```python
from build123d import *

# Parameters (mm, degrees)
SKETCH_1_R          = 20
SKETCH_1_R_2        = 2.015
SKETCH_1_R_3        = 7.5
SKETCH_1_R_4        = 1.6
EXTRUDE_1_DEPTH     = 6
SKETCH_2_W          = 14.17824661
SKETCH_2_H          = 4
CUT_EXTRUDE_1_DEPTH = 10
FILLET_1_R          = 1


with BuildPart() as part:
    # 草图1 → 凸台-拉伸1 (new body)
    with BuildSketch(Plane(origin=(0, 0, 0), x_dir=(1, 0, 0), z_dir=(0, 1, 0))):
        with Locations(Location((0, 0, 0), (0, 0, 270))):
            Circle(SKETCH_1_R)
        with Locations(Location((0, -12.15, 0), (0, 0, 270))):
            Circle(SKETCH_1_R_2, mode=Mode.SUBTRACT)
        with Locations(Location((10.522208656, 6.075, 0), (0, 0, 270))):
            Circle(SKETCH_1_R_2, mode=Mode.SUBTRACT)
        with Locations(Location((-10.522208656, 6.075, 0), (0, 0, 270))):
            Circle(SKETCH_1_R_2, mode=Mode.SUBTRACT)
        with Locations(Location((0, 0, 0), (0, 0, 270))):
            Circle(SKETCH_1_R_3, mode=Mode.SUBTRACT)
        with Locations(Location((-11.691342951, -6.75, 0), (0, 0, 270))):
            Circle(SKETCH_1_R_4, mode=Mode.SUBTRACT)
        with Locations(Location((11.691342951, -6.75, 0), (0, 0, 270))):
            Circle(SKETCH_1_R_4, mode=Mode.SUBTRACT)
        with Locations(Location((0, 13.5, 0), (0, 0, 270))):
            Circle(SKETCH_1_R_4, mode=Mode.SUBTRACT)
    extrude(amount=EXTRUDE_1_DEPTH)

    # 草图2 → 切除-拉伸1 (cut)
    with BuildSketch(Plane(origin=(0, 6, 0), x_dir=(1, 0, 0), z_dir=(0, 1, 0))):
        with Locations((20.089123305, 0)):
            Rectangle(SKETCH_2_W, SKETCH_2_H)
    extrude(amount=-CUT_EXTRUDE_1_DEPTH, mode=Mode.SUBTRACT)

    # 圆角1
    fillet_1_edges = [part.edges().sort_by_distance(p)[0] for p in [
        (13, 3, 2),
        (19.899748742, 3, -2),
        (13, 3, -2),
        (19.899748742, 3, 2),
    ]]
    fillet(fillet_1_edges, radius=FILLET_1_R)


solid = part.part
```
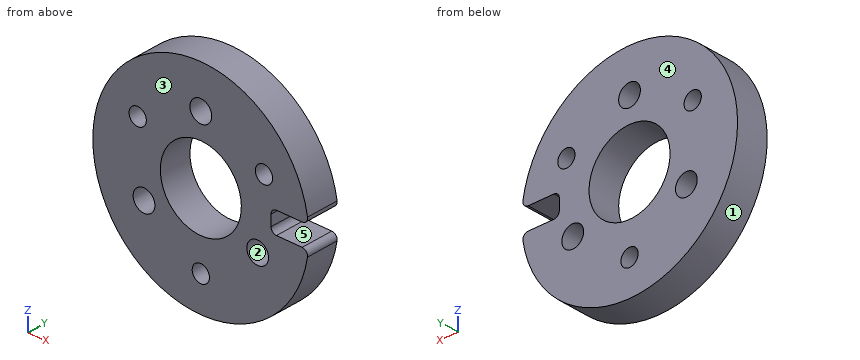
Work out the finished part from the listing and answer in its coordinate system (mm). Face numbers are marked on the shaded views. A direction names the side the tool comes from. Round coordinates to 2 decimals unless told otherwise and drop trailing zeros. Loops run counter-clockwise (first coordinate to the right, second up) from the corner with the lowest first, then second, coordinate; pieces in that order, holes last. Notation, with made-up numbers: M 85,56.25 L 136,56.25 A15 cw 136,63.25 Z; hole C 40,-34 d8. An arc over 180 degrees is marked long. One line per question, with ' | ' between items.
Q1. Find section B-B, the plane x = 0. Give the vertices of the cut face in (y, z) (3 decimals).
Conclusion:
outline: M 0,-20 L 6,-20 L 6,-15.1 L 0,-15.1 Z; M 0,-11.9 L 6,-11.9 L 6,-7.5 L 0,-7.5 Z; M 0,7.5 L 6,7.5 L 6,10.135 L 0,10.135 Z; M 0,14.165 L 6,14.165 L 6,20 L 0,20 Z
Q2. A tool of negligible diameter and unlimited length cuts with its end or side. For the marked faces 4 and 5, from which of +Z, -Z, +X, -X, +Y, -Y can it reach the whole face along a straight path? Write none if from no direction.
Conclusion:
face 4: +Z, -Z, +X, -X, +Y | face 5: +X, +Y, -Y
Q3. Find section D-D, the plane x = -4. Give the vertices of the cut face in (y, z), then the cut area to 3 significant figures.
Conclusion:
outline: M 0,-19.6 L 6,-19.6 L 6,-6.34 L 0,-6.34 Z; M 0,6.34 L 6,6.34 L 6,19.6 L 0,19.6 Z | area: 159 mm2
Q4. Each of these flat-tipped pins is pushed along its axis until it touches: pin 1 Ø3 at (y, z) = (2.5, 11.5) entering from -X; pin 2 Ø1 at (x, z) = (-15.5, 14) entering from -Y; pin 3 Ø3 at (x, z) = (1, -13.5) entering from +Y; pin 4 Ø1 at (x, y) = (-10, 2) entering from -Z. Where does it stop, or does it pass through?
Conclusion:
pin 1: stops at x = -17.32 | pin 2: passes through | pin 3: stops at y = 6 | pin 4: stops at z = -17.6
Q5. Find section A-A, the plane z = 0. Give the vertices of the cut face in (x, y), then the cut area to 3 significant figures.
Conclusion:
outline: M -20,0 L -7.5,0 L -7.5,6 L -20,6 Z; M 7.5,0 L 13,0 L 13,6 L 7.5,6 Z | area: 108 mm2
Q6. Find section C-C, the plane z = 6.75. Give the vertices of the cut face in (x, y).
Conclusion:
outline: M -18.83,0 L -13.29,0 L -13.29,6 L -18.83,6 Z; M -10.09,0 L -3.27,0 L -3.27,6 L -10.09,6 Z; M 3.27,0 L 10.09,0 L 10.09,6 L 3.27,6 Z; M 13.29,0 L 18.83,0 L 18.83,6 L 13.29,6 Z
Q7. The mould has two halves that part along Z. Classify the marked faces 1, 2 and 3: +Z half, -Z half, draft (parallel to the pull), parting line (faces both ways), or undercut.
Conclusion:
face 1: parting line | face 2: undercut | face 3: draft
Q8. Consider line 1 along X through (y, z) = (4.1, 6.75); line 2 along Z through (x, y) = (11.5, 3.95); line 3 along X through (y, z) = (4.35, -3). Determine where each line is inside the solid, lowest interval first. Write a range as from..to.
Conclusion:
line 1: x = -18.83..-13.29, -10.09..-3.27, 3.27..10.09, 13.29..18.83 | line 2: z = -16.36..-7.84, -4.31..5.16, 8.34..16.36 | line 3: x = -19.77..-6.87, 6.87..19.76
